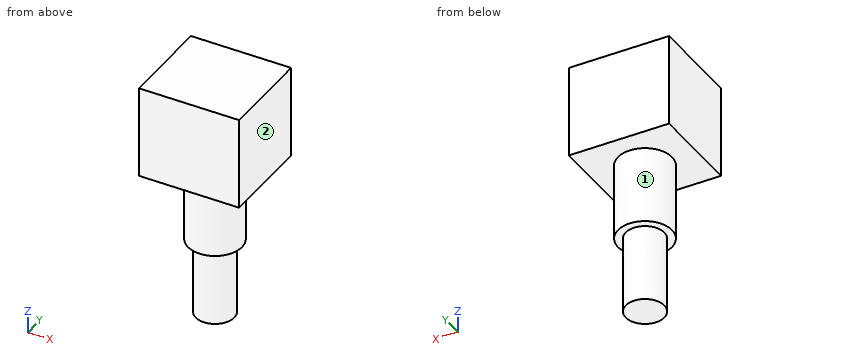
from build123d import *

# Parameters (mm, degrees)
SKETCH029_R             = 3.5
PAD029_DEPTH            = 10
SKETCH030_R             = 2.5
PAD030_DEPTH            = 10
SKETCH031_W             = 13
SKETCH031_H             = 12
PAD031_DEPTH            = 12
BODY011_PLACEMENT_ANGLE = 180


with BuildPart() as part:
    # Sketch029 → Pad029 (new body)
    with BuildSketch(Plane.XY):
        Circle(SKETCH029_R)
    extrude(amount=PAD029_DEPTH)

    # Sketch030 (on Face3 of Pad029) → Pad030 (join)
    with BuildSketch(Plane.XY.offset(10)):
        Circle(SKETCH030_R)
    extrude(amount=PAD030_DEPTH)

    # Sketch031 (on Face2 of Pad030) → Pad031 (join)
    with BuildSketch(Plane(origin=(0, 0, 0), x_dir=(1, 0, 0), z_dir=(0, 0, -1))):
        Rectangle(SKETCH031_W, SKETCH031_H)
    extrude(amount=PAD031_DEPTH)


with BuildPart() as part_1:
    # Body011 placement: moved
    add(part.part.moved(Location((-26, 13.5, 1))).rotate(Axis((-26, 13.5, 1), (0, 1, 0)), BODY011_PLACEMENT_ANGLE))


solid = part_1.part
Could you check a few things on this model? Use its own coordinates, in mm. Face numbers are marked on the shaded views. A direction names the side the tool comes from. Give positions to 0.01 mm unless a question says otherwise; leave off trailing zeros. Order: outer loops, then holes, each group sorted by start corner. A loop starts at its lowest first (then second) coordinate and runs counter-clockwise, first axis right, second up. Notation, with made-up numbers: (53, 15) - (89, 15) arc R13 ccw to (89, 25) - close; hole circle Ø2 at (-16, 58.5). An arc over 180 degrees is marked (long way). One line per question, with ' | ' between items. Start each with the question number.
Item 1: I want a section at C-C on z = -3. Write out the boundary of the cut face in (x, y), then the cut area to 3 significant figures.
Item 2: I want a section at D-D on y = 10.5. Write out the boundary of the cut face in (x, z).
Item 3: I'm going to push flat-ended pins straight in: pin 1 Ø1.5 at (x, z) = (-26.5, -5.5) entering from +Y; pin 2 Ø3 at (y, z) = (17, -13) entering from +X; pin 3 Ø6 at (y, z) = (13.5, -4) entering from -X. Where does each tip first touch, or does it pass through?
Item 4: I want a section at A-A on y = 13.5. Write out the boundary of the cut face in (x, z).
Item 5: For the marked faces 1 and 2, which set-ups out of +Z, -Z, +X, -X, +Y, -Y let a thin tool reach every point of the face, with its end or its side?
Item 6: I want a section at B-B on x = -26. Write out the boundary of the cut face in (y, z), then the cut area to 3 significant figures.
Item 7: I need wall thicknesses on probe 1 along Z at (x, y) = (-25.25, 16); probe 2 along Z at (x, y) = (-20, 8.25); probe 3 along X at (y, z) = (13.75, -4). Which ranges of each line are inside material? Lowest first, please. Write a range as [from, to].
Verdict:
1) outline: circle Ø7 at (-26, 13.5) | area: 38.5 mm^2
2) outline: (-32.5, 1) - (-27.8, 1) - (-27.8, -9) - (-24.2, -9) - (-24.2, 1) - (-19.5, 1) - (-19.5, 13) - (-32.5, 13) - close
3) pin 1: y = 17 | pin 2: x = -24.5 | pin 3: x = -29.5
4) outline: (-32.5, 1) - (-29.5, 1) - (-29.5, -9) - (-28.5, -9) - (-28.5, -19) - (-23.5, -19) - (-23.5, -9) - (-22.5, -9) - (-22.5, 1) - (-19.5, 1) - (-19.5, 13) - (-32.5, 13) - close
5) face 1: -Z | face 2: +Z, -Z, +X, +Y, -Y
6) outline: (7.5, 1) - (10, 1) - (10, -9) - (11, -9) - (11, -19) - (16, -19) - (16, -9) - (17, -9) - (17, 1) - (19.5, 1) - (19.5, 13) - (7.5, 13) - close | area: 264 mm^2
7) probe 1: [-9, 13] | probe 2: [1, 13] | probe 3: [-29.49, -22.51]
